Could you check a few things on this drawing? It's one solid part, dimensions in mm from its lowest x, y, z. Coordinates: 2 decimals unless noted, no trailing zeros. Write each loop counter-clockwise with the first axis right and the second up, starting at its lowest first coordinate (ties: lowest second). Pieces come first, ordered by that corner, then holes.
Item 1: Please list where these lines run through material, in increasing order: line 1 (X direction, y = 73.5, z = 2); line 2 (Y direction, x = 43, z = 1.85) (1 decimal); line 3 (Y direction, x = 43.75, z = 1.9).
Item 2: I'm going to push flat-ended pins straight in: P1, Ø2, axis at x = 20.5, y = 24, coming from the -Z side; P2, Ø2, axis at x = 15.75, y = 73.5, coming from the +Z side. Where does each tip first touch, or does it pass through?
Item 3: I want a section at D-D (z = 1). Count the separate pieces of the cut face and the enclosed holes in it, and give its area (3 significant figures).
Item 4: I want a section at A-A (y = 73.5). Please give me the cut outline in (x, z).
Item 5: I want a section at B-B (x = 23). Please give me the cut outline in (y, z).
Item 6: I want a section at C-C (y = 43). Please give me the cut outline in (x, z).
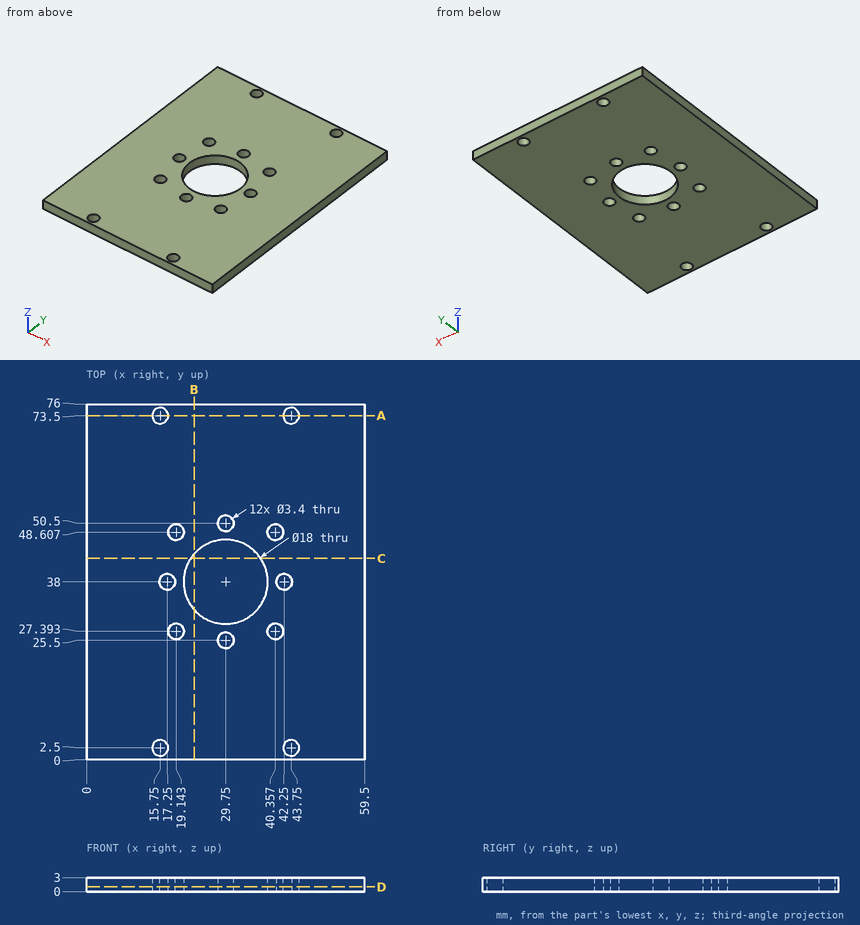
Answer:
1. line 1: x = 0 to 14.05, 17.45 to 42.05, 45.45 to 59.5
1. line 2: y = 0 to 1, 4 to 36.5, 39.5 to 72, 75 to 76
1. line 3: y = 0 to 0.8, 4.2 to 37.2, 38.8 to 71.8, 75.2 to 76
2. P1: stops at z = 0
2. P2: passes through
3. separate pieces: 1
3. enclosed holes: 13
3. area: 4,160 mm2
4. outline: (0, 0) - (14.05, 0) - (14.05, 3) - (0, 3) - close; (17.45, 0) - (42.05, 0) - (42.05, 3) - (17.45, 3) - close; (45.45, 0) - (59.5, 0) - (59.5, 3) - (45.45, 3) - close
5. outline: (0, 0) - (32.05, 0) - (32.05, 3) - (0, 3) - close; (43.95, 0) - (76, 0) - (76, 3) - (43.95, 3) - close
6. outline: (0, 0) - (22.27, 0) - (22.27, 3) - (0, 3) - close; (37.23, 0) - (59.5, 0) - (59.5, 3) - (37.23, 3) - close
